Build history of the part. All positions in model axes, mm. A direction names the side the tool comes from. Round coordinates to 2 decimals unless told otherwise and drop trailing zeros. Write each loop counter-clockwise with the first axis right and the second up, starting at its lowest first coordinate (ties: lowest second). Pieces come first, ordered by that corner, then holes. Notation, with made-up numbers: (50.5, -6.5) - (102.5, -6.5) arc R17 cw to (102.5, 5.5) - close; hole circle Ø11 at (82.5, 13). An arc over 180 degrees is marked (long way). Answer as a JSON object with one key per item and string values. Group by question number.
Item 1: Two-plate mould, pull along Z, no slides. Class faces 1 (the flat face through (-15.453, -0.14, -334.535)), 2 (the flat face through (-25, 0, -190)), 3 (the flat face through (0, 0, -380)): +Z half, -Z half, draft (parallel to the pull), parting line (faces both ways), or undercut.
Item 2: Probe line 1 (X direction, y = -5.75, z = -224.5); line 2 (X direction, y = 2.5, z = -280); line 3 (X direction, y = 1.75, z = -217). List the from-to ranges inside material, lowest first. Write a range as from..to.
Item 3: Slice it at A-A, the plane y = 5. List the corners of the cut face in (x, z), then the cut area to 3 significant figures.
Item 4: Flat gauge pin, fed straight in: pin 1 (10 mm diameter, centred on y = 1, z = -155, fed in from -X). Where does the tip first touch, or does it go through?
Item 5: Which spindle directions (+Z, -Z, +X, -X, +Y, -Y) get a long thin tool onto all of the face, cutting with end or side? Do faces 4 (the cylindrical face through (8, 0, -160)), 5 (the flat face through (-15.453, 0.14, -345.535)). Say none if no direction does.
from build123d import *

# Parameters (mm, degrees)
SKETCH1_W           = 50
SKETCH1_H           = 20
BOSS_EXTRUDE1_DEPTH = 380
SKETCH2_R           = 8
CUT_EXTRUDE1_DEPTH  = 21
CUT_EXTRUDE2_REACH  = 52


with BuildPart() as part:
    # Sketch1 → Boss-Extrude1 (new body)
    with BuildSketch(Plane.XY):
        Rectangle(SKETCH1_W, SKETCH1_H)
    extrude(amount=-BOSS_EXTRUDE1_DEPTH)

    # Sketch2 → Cut-Extrude1 (cut, through all)
    with BuildSketch(Plane(origin=(0, 10, 0), x_dir=(1, 0, 0), z_dir=(0, 1, 0))):
        with Locations((0, 40)):
            Circle(SKETCH2_R)
        with Locations((0, 100)):
            Circle(SKETCH2_R)
        with Locations((0, 160)):
            Circle(SKETCH2_R)
        with Locations((0, 220)):
            Circle(SKETCH2_R)
        with Locations((0, 280)):
            Circle(SKETCH2_R)
        with Locations((0, 340)):
            Circle(SKETCH2_R)
    extrude(amount=-CUT_EXTRUDE1_DEPTH, mode=Mode.SUBTRACT)

    # Sketch3 → Cut-Extrude2 (cut, up to next)
    with BuildSketch(Plane.ZY.offset(25), mode=Mode.PRIVATE) as cut_extrude2_sk1:
        Polygon((-348, 10), (-343, -10), (-337, -10), (-332, 10), align=None)
    cut_extrude2_tool1 = extrude(cut_extrude2_sk1.sketch, amount=-CUT_EXTRUDE2_REACH, mode=Mode.PRIVATE) & part.part
    add(cut_extrude2_tool1.solids().sort_by_distance((-25, 1.515152, -340))[0], mode=Mode.SUBTRACT)
    # Sketch3 → Cut-Extrude2 (cut, up to next)
    with BuildSketch(Plane.ZY.offset(25), mode=Mode.PRIVATE) as cut_extrude2_sk2:
        Polygon((-288, 10), (-283, -10), (-277, -10), (-272, 10), align=None)
    cut_extrude2_tool2 = extrude(cut_extrude2_sk2.sketch, amount=-CUT_EXTRUDE2_REACH, mode=Mode.PRIVATE) & part.part
    add(cut_extrude2_tool2.solids().sort_by_distance((-25, 1.515152, -280))[0], mode=Mode.SUBTRACT)
    # Sketch3 → Cut-Extrude2 (cut, up to next)
    with BuildSketch(Plane.ZY.offset(25), mode=Mode.PRIVATE) as cut_extrude2_sk3:
        Polygon((-228, 10), (-223, -10), (-217, -10), (-212, 10), align=None)
    cut_extrude2_tool3 = extrude(cut_extrude2_sk3.sketch, amount=-CUT_EXTRUDE2_REACH, mode=Mode.PRIVATE) & part.part
    add(cut_extrude2_tool3.solids().sort_by_distance((-25, 1.515152, -220))[0], mode=Mode.SUBTRACT)
    # Sketch3 → Cut-Extrude2 (cut, up to next)
    with BuildSketch(Plane.ZY.offset(25), mode=Mode.PRIVATE) as cut_extrude2_sk4:
        Polygon((-168, 10), (-163, -10), (-157, -10), (-152, 10), align=None)
    cut_extrude2_tool4 = extrude(cut_extrude2_sk4.sketch, amount=-CUT_EXTRUDE2_REACH, mode=Mode.PRIVATE) & part.part
    add(cut_extrude2_tool4.solids().sort_by_distance((-25, 1.515152, -160))[0], mode=Mode.SUBTRACT)
    # Sketch3 → Cut-Extrude2 (cut, up to next)
    with BuildSketch(Plane.ZY.offset(25), mode=Mode.PRIVATE) as cut_extrude2_sk5:
        Polygon((-108, 10), (-103, -10), (-97, -10), (-92, 10), align=None)
    cut_extrude2_tool5 = extrude(cut_extrude2_sk5.sketch, amount=-CUT_EXTRUDE2_REACH, mode=Mode.PRIVATE) & part.part
    add(cut_extrude2_tool5.solids().sort_by_distance((-25, 1.515152, -100))[0], mode=Mode.SUBTRACT)
    # Sketch3 → Cut-Extrude2 (cut, up to next)
    with BuildSketch(Plane.ZY.offset(25), mode=Mode.PRIVATE) as cut_extrude2_sk6:
        Polygon((-48, 10), (-43, -10), (-37, -10), (-32, 10), align=None)
    cut_extrude2_tool6 = extrude(cut_extrude2_sk6.sketch, amount=-CUT_EXTRUDE2_REACH, mode=Mode.PRIVATE) & part.part
    add(cut_extrude2_tool6.solids().sort_by_distance((-25, 1.515152, -40))[0], mode=Mode.SUBTRACT)


solid = part.part
Geometry says:
{
 "1": {"face 1": "undercut", "face 2": "draft", "face 3": "-Z half"},
 "2": {"line 1": "x = -25..-6.61, 6.61..25", "line 2": "x = 8..25", "line 3": "x = 7.42..25"},
 "3": {"outline": "(-25, -380) - (25, -380) - (25, 0) - (-25, 0) - (-25, -33.25) - (-4.29, -33.25) arc R8 cw (long way) to (-4.29, -46.75) - (-25, -46.75) - (-25, -93.25) - (-4.29, -93.25) arc R8 cw (long way) to (-4.29, -106.75) - (-25, -106.75) - (-25, -153.25) - (-4.29, -153.25) arc R8 cw (long way) to (-4.29, -166.75) - (-25, -166.75) - (-25, -213.25) - (-4.29, -213.25) arc R8 cw (long way) to (-4.29, -226.75) - (-25, -226.75) - (-25, -273.25) - (-4.29, -273.25) arc R8 cw (long way) to (-4.29, -286.75) - (-25, -286.75) - (-25, -333.25) - (-4.29, -333.25) arc R8 cw (long way) to (-4.29, -346.75) - (-25, -346.75) - close", "area": "16,300 mm^2"},
 "4": {"pin 1": "stops at x = -25"},
 "5": {"face 4": "+Y, -Y", "face 5": "-X, +Y"}
}
